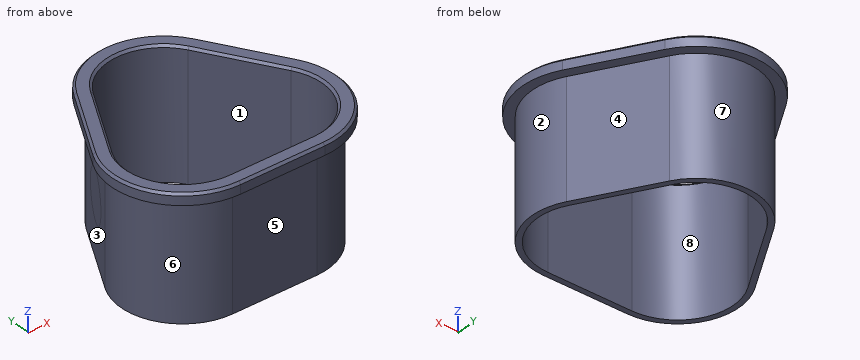
from build123d import *

# Parameters (mm, degrees)
F1_DEPTH      = 25
F2_R          = 4.3
F3_DEPTH      = 3
F3_DEPTH_BACK = 0.65
F5_R          = 40.103887
F6_DEPTH      = 2
F7_R          = 28.872497
F8_DEPTH      = 21
F9_R          = 30.144829
F10_DEPTH     = 25
F11_SIZE      = 0.4


with BuildPart() as f1:
    # F0 (on Top) → F1 (new body)
    with BuildSketch(Plane.XY):
        with BuildLine():
            ThreePointArc((7.679492, -4), (19.803848, 3), (19.803848, 17))
            Line((19.803848, 17), (12.124356, 30.30127))
            ThreePointArc((12.124356, 30.30127), (0, 37.30127), (-12.124356, 30.30127))
            Line((-12.124356, 30.30127), (-19.803848, 17))
            ThreePointArc((-19.803848, 17), (-19.803848, 3), (-7.679492, -4))
            Line((-7.679492, -4), (0, -4))
            Line((0, -4), (7.679492, -4))
        make_face()
        with BuildLine():
            Line((7.679492, 0), (0, 0))
            Line((0, 0), (-7.679492, 0))
            ThreePointArc((-7.679492, 0), (-16.339746, 5), (-16.339746, 15))
            Line((-16.339746, 15), (-8.660254, 28.30127))
            ThreePointArc((-8.660254, 28.30127), (0, 33.30127), (8.660254, 28.30127))
            Line((8.660254, 28.30127), (16.339746, 15))
            ThreePointArc((16.339746, 15), (16.339746, 5), (7.679492, 0))
        make_face(mode=Mode.SUBTRACT)
    extrude(amount=F1_DEPTH)

    # F2 (on face) → F3 (cut, two sides)
    with BuildSketch(Plane(origin=(-22.214102, 12.825318, 0), x_dir=(-0.5, -0.866025, 0), z_dir=(-0.866025, 0.5, 0))) as f3_sk:
        with Locations((-12.5, 12.5)):
            Circle(F2_R)
    extrude(amount=-F3_DEPTH, mode=Mode.SUBTRACT)
    extrude(f3_sk.sketch, amount=-F3_DEPTH_BACK, mode=Mode.SUBTRACT)

    # F5 (on face) → F6 (cut)
    with BuildSketch(Plane(origin=(0, 0, 0), x_dir=(1, 0, 0), z_dir=(0, 0, -1))):
        with Locations((0, -16.662003)):
            Circle(F5_R)
    extrude(amount=-F6_DEPTH, mode=Mode.SUBTRACT)

    # F7 (on face) → F8 (cut)
    with BuildSketch(Plane(origin=(0, 0, 2), x_dir=(1, 0, 0), z_dir=(0, 0, -1))):
        with Locations((0, -15.382648)):
            Circle(F7_R)
        with BuildLine():
            Line((-9.526279, -28.80127), (-17.205771, -15.5))
            ThreePointArc((-17.205771, -15.5), (-17.205771, -4.5), (-7.679492, 1))
            Line((-7.679492, 1), (7.679492, 1))
            ThreePointArc((7.679492, 1), (17.205771, -4.5), (17.205771, -15.5))
            Line((17.205771, -15.5), (9.526279, -28.80127))
            ThreePointArc((9.526279, -28.80127), (0, -34.30127), (-9.526279, -28.80127))
        make_face(mode=Mode.SUBTRACT)
    extrude(amount=-F8_DEPTH, mode=Mode.SUBTRACT)

    # F9 (on face) → F10 (cut)
    with BuildSketch(Plane.XY.offset(25)):
        with Locations((-0.752793, 11.019209)):
            Circle(F9_R)
        with BuildLine():
            ThreePointArc((-7.679492, -2.75), (-18.721316, 3.625), (-18.721316, 16.375))
            Line((-18.721316, 16.375), (-11.041824, 29.67627))
            ThreePointArc((-11.041824, 29.67627), (0, 36.05127), (11.041824, 29.67627))
            Line((11.041824, 29.67627), (18.721316, 16.375))
            ThreePointArc((18.721316, 16.375), (18.721316, 3.625), (7.679492, -2.75))
            Line((7.679492, -2.75), (-7.679492, -2.75))
        make_face(mode=Mode.SUBTRACT)
    extrude(amount=-F10_DEPTH, mode=Mode.SUBTRACT)

    # F11
    f11_edges = [f1.edges().sort_by_distance(p)[0] for p in [
        (-14.88157, 23.025635, 25),
        (-12.5, 21.650635, 25),
    ]]
    chamfer(f11_edges, length=F11_SIZE)


solid = f1.part
Here's how the part is built. I have some questions about the finished solid (model axes, mm). Face numbers are marked on the shaded views. A direction names the side the tool comes from. Coordinates: 2 decimals unless noted, no trailing zeros. Loops run counter-clockwise (first coordinate to the right, second up) from the corner with the lowest first, then second, coordinate; pieces in that order, holes last. Notation, with made-up numbers: (9.25, -4) -> (53.25, -4) arc R33 ccw to (53.25, 29) -> close; hole circle Ø11 at (53, -19). An arc over 180 degrees is marked (long way). Use one line per item in the form item = value. Start each with the question number.
(1) If we section it at A-A (z = 22): Please give me the cut outline in (x, y).
(2) Will these pins go through, and if not, where does the flat tip stop? pin 1 (1.5 mm diameter, centred on y = 8, z = 16, fed in from -X); pin 2 (5 mm diameter, centred on y = 29.5, z = 12, fed in from -X); pin 3 (6 mm diameter, centred on x = 8, z = 11.5, fed in from +Y).
(3) Please list where these lines run through material, in increasing order: line 1 along X through (y, z) = (10, 4.75); line 2 along Y through (x, z) = (-15, 10.25); line 3 along X through (y, z) = (4, 17.25).
(4) On a 3-axis mill with a long thin cutter (end or side, diameter ignored), from which of +Z, -Z, +X, -X, +Y, -Y can I reach the whole of each face in a straight line? I mean the marked faces 4, 5, 6, 7 and 8. Say none if no direction works.
(5) We'd pull the mould along X, two halves only. Please class the marked faces 1, 2 and 3: pulls with the +X half, pulls with the -X half, needs draft (parallel to the pull), parting line crosses it, or undercut.
Verdict:
q1.outline = (-17.21, 15.5) arc R11 ccw to (-7.68, -1) -> (7.68, -1) arc R11 ccw to (17.21, 15.5) -> (9.53, 28.8) arc R11 ccw to (-9.53, 28.8) -> close; hole (-16.34, 15) arc R10 ccw to (-7.68, 0) -> (7.68, 0) arc R10 ccw to (16.34, 15) -> (8.66, 28.3) arc R10 ccw to (-8.66, 28.3) -> close
q2.pin_1 = -18.61
q2.pin_2 = -10.57
q2.pin_3 = 33.1
q3.line_1 = -18.68 to -17.68, 17.68 to 18.68
q3.line_2 = 1.79 to 3.19, 17.32 to 19.32
q3.line_3 = -16.9 to -15.68, 15.68 to 16.9
q4.face_4 = -Z, +X, +Y
q4.face_5 = -Z, +X, -X, -Y
q4.face_6 = -Z, -X
q4.face_7 = -Z, +Y
q4.face_8 = +Z, -Z
q5.face_1 = undercut
q5.face_2 = pulls with the +X half
q5.face_3 = pulls with the -X half
